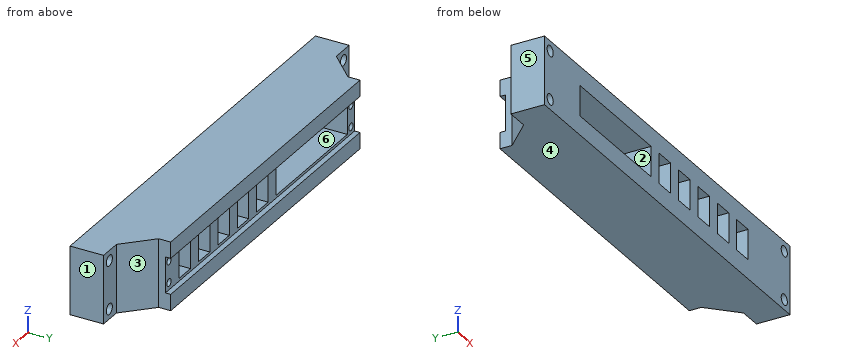
Autodesk Inventor part; units mm, degrees
ref_plane "YZ Plane" through (0, 0, 0) normal (1, 0, 0) x (0, 1, 0)
ref_plane "XZ Plane" through (0, 0, 0) normal (0, 1, 0) x (-1, 0, 0)
ref_plane "XY Plane" through (0, 0, 0) normal (0, 0, 1) x (1, 0, 0)
sketch "Sketch1" plane through (0, 0, 0) normal (0, 1, 0) x (-1, 0, 0)
  line L0 (0, 0) -> (128.5, 0)
  line L1 (128.5, 0) -> (128.5, -20.32)
  line L2 (128.5, -20.32) -> (0, -20.32)
  line L3 (0, -20.32) -> (0, 0)
  dimension "d0" = 20.32
  dimension "d1" = 128.5
extrude "Extrusion1" add sketch "Sketch1" along normal blind 10
sketch "Sketch2" plane through (0, 10, 0) normal (0, 1, 0) x (1, 0, 0)
  line L0 (-128.5, 0) -> (0, 0)
  line L1 (0, 0) -> (0, 20.32)
  line L2 (0, 20.32) -> (-128.5, 20.32)
  line L3 (-128.5, 20.32) -> (-128.5, 0)
  line L4 (-128.5, 0) -> (0, 0)
  line L5 (0, 20.32) -> (-128.5, 20.32)
  line L6 (-14.72, 0) -> (-113.78, 0)
  line L7 (-113.78, 0) -> (-113.78, 20.32)
  line L8 (-113.78, 20.32) -> (-14.72, 20.32)
  line L9 (-14.72, 20.32) -> (-14.72, 0)
  line L10 (-128.5, 20.32) -> (-113.78, 20.32)
  line L11 (-128.5, 20.32) -> (0, 20.32)
  line L12 (-14.72, 20.32) -> (0, 20.32)
  line L13 (-128.5, 10.16) -> (-113.78, 10.16)
  line L14 (-14.72, 10.16) -> (0, 10.16)
  dimension "d19" = 99.06
extrude "Extrusion2" add sketch "Sketch2" along normal blind 10 contours L7 L2 L9 L0
sketch "Sketch3" plane through (0, 10, 0) normal (0, 1, 0) x (1, 0, 0)
  line L0 (-113.78, 0) -> (-113.78, 20.32)
  line L1 (-113.78, 20.32) -> (-128.5, 20.32)
  line L2 (-128.5, 20.32) -> (-128.5, 0)
  line L3 (-128.5, 0) -> (-113.78, 0)
  line L4 (-14.72, 20.32) -> (-14.72, 0)
  line L5 (-14.72, 0) -> (0, 0)
  line L6 (0, 0) -> (0, 20.32)
  line L7 (0, 20.32) -> (-14.72, 20.32)
  line L8 (-113.78, 20.32) -> (-128.5, 20.32)
  line L9 (-128.5, 0) -> (-125.5, 0)
  line L10 (-125.5, 0) -> (-125.5, 20.32)
  line L11 (-125.5, 20.32) -> (-128.5, 20.32)
  line L12 (-128.5, 20.32) -> (-128.5, 0)
  line L13 (-128.5, 20.32) -> (0, 20.32)
  line L14 (0, 0) -> (-3, 0)
  line L15 (-3, 0) -> (-3, 20.32)
  line L16 (-3, 20.32) -> (0, 20.32)
  line L17 (0, 20.32) -> (0, 0)
  line L18 (-125.5, 0) -> (-3, 0)
  line L19 (-3, 0) -> (-3, 3)
  line L20 (-3, 3) -> (-125.5, 3)
  line L21 (-125.5, 3) -> (-125.5, 0)
  line L22 (-125.5, 20.32) -> (-3, 20.32)
  line L23 (-3, 20.32) -> (-3, 17.32)
  line L24 (-3, 17.32) -> (-125.5, 17.32)
  line L25 (-125.5, 17.32) -> (-125.5, 20.32)
  dimension "d8" = 3
  dimension "d9" = 3
  dimension "d10" = 3
  dimension "d11" = 3
hole "Hole1" at (-125.5, 10, -3) at (-125.5, 10, -17.32) at (-3, 10, -17.32) at (-3, 10, -3) direction (0, -1, 0) diameter 3.2 end through all
sketch "Sketch4" plane through (0, 20, 0) normal (0, 1, 0) x (1, 0, 0)
  line L0 (-14.72, 20.32) -> (-14.72, 0)
  line L1 (-14.72, 10.16) -> (-113.78, 10.16)
  line L2 (-113.78, 20.32) -> (-113.78, 0)
  line L3 (-27.88, 5.66) -> (-21.88, 5.66)
  line L4 (-21.88, 5.66) -> (-21.88, 14.66)
  line L5 (-21.88, 14.66) -> (-27.88, 14.66)
  line L6 (-27.88, 14.66) -> (-27.88, 5.66)
  line L7 (-27.88, 5.66) -> (-21.88, 14.66) construction
  line L8 (-21.88, 5.66) -> (-27.88, 14.66) construction
  line L9 (-38.04, 5.66) -> (-32.04, 5.66)
  line L10 (-32.04, 5.66) -> (-32.04, 14.66)
  line L11 (-32.04, 14.66) -> (-38.04, 14.66)
  line L12 (-38.04, 14.66) -> (-38.04, 5.66)
  line L13 (-38.04, 5.66) -> (-32.04, 14.66) construction
  line L14 (-32.04, 5.66) -> (-38.04, 14.66) construction
  line L15 (-48.2, 5.66) -> (-42.2, 5.66)
  line L16 (-42.2, 5.66) -> (-42.2, 14.66)
  line L17 (-42.2, 14.66) -> (-48.2, 14.66)
  line L18 (-48.2, 14.66) -> (-48.2, 5.66)
  line L19 (-48.2, 5.66) -> (-42.2, 14.66) construction
  line L20 (-42.2, 5.66) -> (-48.2, 14.66) construction
  line L21 (-58.36, 5.66) -> (-52.36, 5.66)
  line L22 (-52.36, 5.66) -> (-52.36, 14.66)
  line L23 (-52.36, 14.66) -> (-58.36, 14.66)
  line L24 (-58.36, 14.66) -> (-58.36, 5.66)
  line L25 (-58.36, 5.66) -> (-52.36, 14.66) construction
  line L26 (-52.36, 5.66) -> (-58.36, 14.66) construction
  line L27 (-68.52, 5.66) -> (-62.52, 5.66)
  line L28 (-62.52, 5.66) -> (-62.52, 14.66)
  line L29 (-62.52, 14.66) -> (-68.52, 14.66)
  line L30 (-68.52, 14.66) -> (-68.52, 5.66)
  line L31 (-68.52, 5.66) -> (-62.52, 14.66) construction
  line L32 (-62.52, 5.66) -> (-68.52, 14.66) construction
  line L33 (-78.68, 5.66) -> (-72.68, 5.66)
  line L34 (-72.68, 5.66) -> (-72.68, 14.66)
  line L35 (-72.68, 14.66) -> (-78.68, 14.66)
  line L36 (-78.68, 14.66) -> (-78.68, 5.66)
  line L37 (-78.68, 5.66) -> (-72.68, 14.66) construction
  line L38 (-72.68, 5.66) -> (-78.68, 14.66) construction
  line L39 (-72.68, 14.66) -> (-109.97, 14.66)
  line L40 (-109.97, 14.66) -> (-109.97, 5.66)
  line L41 (-109.97, 5.66) -> (-72.68, 5.66)
  line L42 (-72.68, 5.66) -> (-72.68, 14.66)
  point P0 (-24.88, 10.16)
  point P1 (-35.04, 10.16)
  point P2 (-45.2, 10.16)
  point P3 (-55.36, 10.16)
  point P4 (-65.52, 10.16)
  point P5 (-75.68, 10.16)
  dimension "d22" = 6
  dimension "d23" = 9
  dimension "d24" = 10.16
  dimension "d25" = 6
  dimension "d26" = 9
  dimension "d27" = 10.16
  dimension "d28" = 6
  dimension "d29" = 9
  dimension "d30" = 6
  dimension "d31" = 9
  dimension "d32" = 6
  dimension "d33" = 9
  dimension "d34" = 6
  dimension "d35" = 9
  dimension "d36" = 10.16
  dimension "d37" = 10.16
  dimension "d38" = 10.16
  dimension "d39" = 10.16
  dimension "d41" = 3.81
extrude "Extrusion3" cut sketch "Sketch4" against normal through all
sketch "Sketch5" plane through (0, 20, 0) normal (0, 1, 0) x (1, 0, 0)
  line L0 (-14.72, 0) -> (-14.72, 20.32)
  line L1 (-113.78, 20.32) -> (-113.78, 0)
  line L2 (-14.72, 0) -> (-113.78, 20.32)
  line L3 (-113.78, 0) -> (-14.72, 20.32)
  line L4 (-111.875, 13.335) -> (-111.875, 6.985)
  line L5 (-111.875, 6.985) -> (-16.625, 6.985)
  line L6 (-16.625, 6.985) -> (-16.625, 13.335)
  line L7 (-16.625, 13.335) -> (-111.875, 13.335)
  line L8 (-111.875, 13.335) -> (-16.625, 6.985) construction
  line L9 (-111.875, 6.985) -> (-16.625, 13.335) construction
  point P0 (0, 0)
  point P1 (-64.25, 10.16)
  dimension "d44" = 95.25
  dimension "d45" = 6.35
hole "Hole2" at (-16.625, 20, -13.335) at (-16.625, 20, -6.985) at (-111.875, 20, -13.335) at (-111.875, 20, -6.985) direction (0, -1, 0) diameter 2.2 depth 16 tip angle 118
chamfer "Chamfer1" distance 8 angle 45 2 edges at (-14.72, 10, -10.16) (-113.78, 10, -10.16)
sketch "Sketch6" plane through (0, 20, 0) normal (0, 1, 0) x (1, 0, 0)
  line L0 (-14.72, 0) -> (-14.72, 20.32)
  line L1 (-113.78, 20.32) -> (-121.78, 20.32)
  line L2 (-14.72, 20.32) -> (-113.78, 20.32)
  line L3 (-113.78, 20.32) -> (-113.78, 15.49)
  line L4 (-113.78, 15.49) -> (-14.72, 15.49)
  line L5 (-14.72, 15.49) -> (-14.72, 20.32)
  line L6 (-113.78, 0) -> (-14.72, 0)
  line L7 (-14.72, 0) -> (-14.72, 4.83)
  line L8 (-14.72, 4.83) -> (-113.78, 4.83)
  line L9 (-113.78, 4.83) -> (-113.78, 0)
  point P0 (0, 0)
  dimension "d56" = 10.66
extrude "Extrusion4" add sketch "Sketch6" along normal blind 1.6
properties part number "OttosDIY_Testing"
The listing builds one solid part. Answer for the finished solid, in the listing's coordinates (mm). Face numbers are marked on the shaded views. A direction names the side the tool comes from. Round coordinates to 2 decimals unless told otherwise and drop trailing zeros. Order: outer loops, then holes, each group sorted by start corner. A loop starts at its lowest first (then second) coordinate and runs counter-clockwise, first axis right, second up. Notation, with made-up numbers: (34.25, 80) -> (39.25, 80) arc R20 ccw to (39.25, 107) -> close; hole circle Ø1 at (-28.75, 45). An arc over 180 degrees is marked (long way). One line per item, written item: value.
Item 1: For a pull along X with two mould halves and no side action, classify the marked faces 3, 4, 5 and 6 as released by +X, released by -X, zero draft, split by the parting line, or undercut.
Taken from the geometry:
face 3: released by +X
face 4: zero draft
face 5: released by -X
face 6: undercut
Item 2: For the marked faces 1 and 2, determine the directions among +Z, -Z, +X, -X, +Y, -Y from which every point of the face is accessible in a straight line to the end or side of a thin tool.
Taken from the geometry:
face 1: +Z, -Z, +X, +Y, -Y
face 2: +Y, -Y
Item 3: Find section A-A, the plane x = -125.5. Give the vertices of the cut face in (y, z).
Taken from the geometry:
outline: (0, -20.32) -> (10, -20.32) -> (10, -18.92) -> (0, -18.92) -> close; (0, -15.72) -> (10, -15.72) -> (10, -4.6) -> (0, -4.6) -> close; (0, -1.4) -> (10, -1.4) -> (10, 0) -> (0, 0) -> close
Item 4: Straight lines are drawn through the part: L1, parallel to X at y = 7.25, z = -3; L2, parallel to Z at x = -3, y = 3.75; L3, parallel to Z at x = -86, y = 9. For each, find the intervals that lie inside material, in ascending order.
Taken from the geometry:
L1: x = -128.5 to -127.1, -123.9 to -4.6, -1.4 to 0
L2: z = -20.32 to -18.92, -15.72 to -4.6, -1.4 to 0
L3: z = -20.32 to -14.66, -5.66 to 0
Item 5: Find section B-B, the plane z = -17.32. Give the vertices of the cut face in (x, y).
Taken from the geometry:
outline: (-128.5, 0) -> (-127.1, 0) -> (-127.1, 10) -> (-128.5, 10) -> close; (-123.9, 0) -> (-4.6, 0) -> (-4.6, 10) -> (-6.72, 10) -> (-14.72, 18) -> (-14.72, 21.6) -> (-113.78, 21.6) -> (-113.78, 18) -> (-121.78, 10) -> (-123.9, 10) -> close; (-1.4, 0) -> (0, 0) -> (0, 10) -> (-1.4, 10) -> close
Item 6: Find section C-C, the plane x = -60. Give the vertices of the cut face in (y, z), then the cut area to 3 significant figures.
Taken from the geometry:
outline: (0, -20.32) -> (21.6, -20.32) -> (21.6, -15.49) -> (20, -15.49) -> (20, -4.83) -> (21.6, -4.83) -> (21.6, 0) -> (0, 0) -> close
area: 422 mm2
Item 7: Given P1, Ø12, axis at x = -20.5, y = 18, coming from the +Z side; P2, Ø1.9, axis at x = -3, z = -17.32, coming from the -Y side; P3, Ø12, axis at y = 18.5, z = -11, coming from the -X side; P4, Ø3.5, axis at x = -16.625, z = -6.985, coming from the +Y side, each flat-ended and moving along its own axis, determine where each tip first touches the part or whether it passes through.
Taken from the geometry:
P1: stops at z = 0
P2: passes through
P3: stops at x = -119.28
P4: stops at y = 20
Item 8: Find section D-D, the plane y = 5.75. State how many separate pieces and enclosed holes the cut face has, then the cut area to 3 significant figures.
Taken from the geometry:
separate pieces: 1
enclosed holes: 14
area: 1,960 mm2
